from build123d import *

# Parameters (mm, degrees)
SCHIZZO1_W                   = 70
SCHIZZO1_H                   = 18
ESTRUSIONE_ESTRUSIONE1_DEPTH = 10
RACCORDO1_R                  = 2.5
RACCORDO2_R                  = 2.5
RACCORDO3_R                  = 2.5
RACCORDO4_R                  = 2.5
FORO_PER_VITE_5_16_3_D       = 5.999999938
SCHIZZO6_W                   = 28
SCHIZZO6_H                   = 15
ESTRUSIONE_ESTRUSIONE2_DEPTH = 3
FORO_PER_VITE_M4_1_D         = 5.5
SCHIZZO12_W                  = 22.4
SCHIZZO12_H                  = 2
ESTRUSIONE_ESTRUSIONE3_DEPTH = 23.65
SCHIZZO13_R                  = 1.75
TAGLIO_ESTRUSIONE1_DEPTH     = 23.75


with BuildPart() as part:
    # Schizzo1 → Estrusione-Estrusione1 (new body)
    with BuildSketch(Plane(origin=(0, 0, 0), x_dir=(1, 0, 0), z_dir=(0, 1, 0))):
        Rectangle(SCHIZZO1_W, SCHIZZO1_H)
    extrude(amount=ESTRUSIONE_ESTRUSIONE1_DEPTH)

    # Raccordo1
    raccordo1_edges = [part.edges().sort_by_distance(p)[0] for p in [
        (0, 10, -9),
    ]]
    fillet(raccordo1_edges, radius=RACCORDO1_R)

    # Raccordo2
    raccordo2_edges = [part.edges().sort_by_distance(p)[0] for p in [
        (0, 10, 9),
    ]]
    fillet(raccordo2_edges, radius=RACCORDO2_R)

    # Raccordo3
    raccordo3_edges = [part.edges().sort_by_distance(p)[0] for p in [
        (0, 0, -9),
    ]]
    fillet(raccordo3_edges, radius=RACCORDO3_R)

    # Raccordo4
    raccordo4_edges = [part.edges().sort_by_distance(p)[0] for p in [
        (0, 0, 9),
    ]]
    fillet(raccordo4_edges, radius=RACCORDO4_R)

    # Foro per Vite 5/16-3 (through all)
    with Locations(Plane(origin=(30, 5, -9), x_dir=(-1, 0, 0), z_dir=(0, 0, -1))):
        with Locations((0, 0)):
            Hole(FORO_PER_VITE_5_16_3_D / 2)

    # Schizzo6 → Estrusione-Estrusione2 (add)
    with BuildSketch(Plane.ZY.offset(35)):
        with Locations((0, 5)):
            Rectangle(SCHIZZO6_W, SCHIZZO6_H)
    extrude(amount=ESTRUSIONE_ESTRUSIONE2_DEPTH)

    # Foro per Vite M4-1 (through all)
    with Locations(Plane.ZY.offset(38)):
        with Locations((0, 5)):
            Hole(FORO_PER_VITE_M4_1_D / 2)

    # Schizzo12 → Estrusione-Estrusione3 (add)
    with BuildSketch(Plane.ZY.offset(38)):
        with Locations((0, 0.05)):
            Rectangle(SCHIZZO12_W, SCHIZZO12_H)
    extrude(amount=ESTRUSIONE_ESTRUSIONE3_DEPTH)

    # Schizzo13 → Taglio-Estrusione1 (cut)
    with BuildSketch(Plane.XZ.offset(0.95)):
        with Locations(Location((-55.5, 0, 0), (0, 0, 270))):
            Circle(SCHIZZO13_R)
    extrude(amount=-TAGLIO_ESTRUSIONE1_DEPTH, mode=Mode.SUBTRACT)


solid = part.part
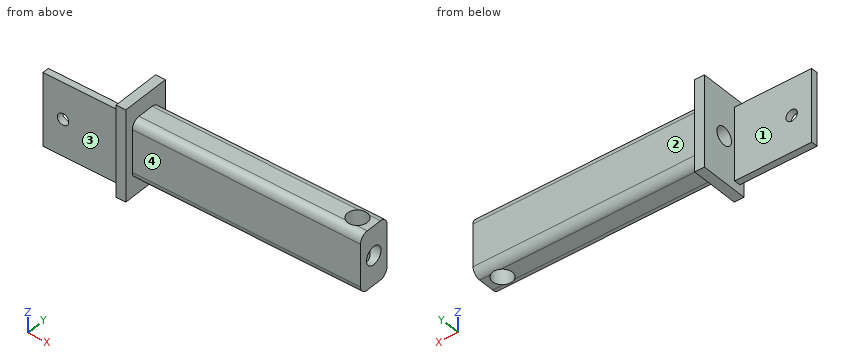
Verification items for the finished model (mm, model axes). Face numbers are marked on the shaded views. A direction names the side the tool comes from. Give positions to 0.01 mm unless a question says otherwise; leave off trailing zeros. Order: outer loops, then holes, each group sorted by start corner. A loop starts at its lowest first (then second) coordinate and runs counter-clockwise, first axis right, second up. Notation, with made-up numbers: M -24,83.5 L 19,83.5 A22 ccw 19,93.5 Z; hole C 28.5,-32.5 d9. An arc over 180 degrees is marked long. Use one line per item in the form item = value. Start each with the question number.
Q1. Scan lines: line 1 along Z through (x, y) = (-17, 5); line 2 along Y through (x, z) = (32.5, 0); line 3 along X through (y, z) = (-0.3, 0). Record each from-to range of solid material in increasing order. Write a range as [from, to].
Q2. Section check A-A (y = 5). Enter the section's corners in (x, z), then the cut area to 4 significant figures.
Q3. Section check D-D (x = 30). Enter the section's corners in (y, z), then the cut area to 3 significant figures.
Q4. Access from +Z, -Z, +X, -X, +Y, -Y to the whole of each face (thin tool, end or side, straight path). Record for the marked faces 1, 2, 3 and 4.
Q5. Go/stop test with flat-tipped pins: pin 1 Ø1 at (x, y) = (4, 0) entering from -Z; pin 2 Ø4 at (x, z) = (-15.5, -0.5) entering from -Y; pin 3 Ø3.5 at (y, z) = (5, 0) entering from +X; pin 4 Ø5 at (x, z) = (-19.5, 0.5) entering from +Y. Record where each tip stops, or that it passes through.
Q6. Section check C-C (z = -4). Enter the section's corners in (x, y), then the cut area to 3 significant figures.
Q7. Section check B-B (z = 0). Enter the section's corners in (x, y), then the cut area to 3 significant figures.
Evaluation:
q1.line_1 = [-9, -2.75], [2.75, 9]
q1.line_2 = [0, 2.25], [7.75, 10]
q1.line_3 = [-61.65, -57.25], [-53.75, -35]
q2.outline = M -38,-14 L -35,-14 L -35,-9 L 27,-9 L 27,-2.75 L -38,-2.75 Z; M -38,2.75 L 27,2.75 L 27,9 L -35,9 L -35,14 L -38,14 Z; M 33,-9 L 35,-9 L 35,-2.75 L 33,-2.75 Z; M 33,2.75 L 35,2.75 L 35,9 L 33,9 Z
q2.area = 867.5 mm2
q3.outline = M 0,-6.5 A2.5 ccw 2,-8.95 L 2,8.95 A2.5 ccw 0,6.5 Z; M 8,-8.95 A2.5 ccw 10,-6.5 L 10,6.5 A2.5 ccw 8,8.95 Z
q3.area = 66.7 mm2
q4.face_1 = +Z, -Z, -X, +Y
q4.face_2 = +Z, -Z, +X, +Y
q4.face_3 = +Z, -Z, -X, -Y
q4.face_4 = +Z, -Z, +X, -Y
q5.pin_1 = -8
q5.pin_2 = 0
q5.pin_3 = through
q5.pin_4 = 10
q6.outline = M -61.65,-0.95 L -38,-0.95 L -38,-2.5 L -35,-2.5 L -35,0 L 35,0 L 35,10 L -35,10 L -35,12.5 L -38,12.5 L -38,1.05 L -61.65,1.05 Z; hole C 30,5 d6
q6.area = 764 mm2
q7.outline = M -61.65,-0.95 L -57.25,-0.95 L -57.25,1.05 L -61.65,1.05 Z; M -53.75,-0.95 L -38,-0.95 L -38,-2.5 L -35,-2.5 L -35,0 L 35,0 L 35,2.25 L 31.2,2.25 A3 cw 28.8,2.25 L -38,2.25 L -38,1.05 L -53.75,1.05 Z; M -38,7.75 L 28.8,7.75 A3 cw 31.2,7.75 L 35,7.75 L 35,10 L -35,10 L -35,12.5 L -38,12.5 Z
q7.area = 383 mm2
